Here's how the part is built. I have some questions about the finished solid (model axes, mm). Face numbers are marked on the shaded views. A direction names the side the tool comes from. Coordinates: 2 decimals unless noted, no trailing zeros. Write each loop counter-clockwise with the first axis right and the second up, starting at its lowest first coordinate (ties: lowest second). Pieces come first, ordered by that corner, then holes.
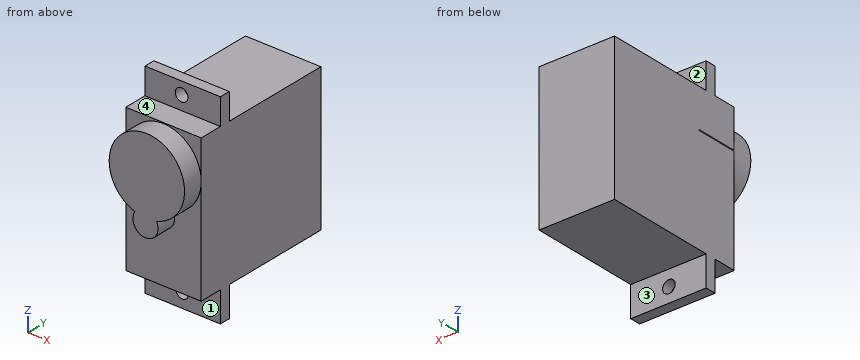
```python
from build123d import *

# Parameters (mm, degrees)
CYLINDER036_R             = 6
CYLINDER036_DEPTH         = 10
CYLINDER032_R             = 1
CYLINDER032_DEPTH         = 10
CYLINDER034_R             = 1
CYLINDER034_DEPTH         = 10
BOX003_W                  = 23
BOX003_H                  = 12
BOX003_DEPTH              = 23
BOX004_W                  = 32
BOX004_H                  = 12
BOX004_DEPTH              = 1.7
CYLINDER035_R             = 2
CYLINDER035_DEPTH         = 10
FUSION005_PITCH_ANGLE     = 90
FUSION005_PLACEMENT_ANGLE = -90


with BuildPart() as cylinder036:
    # Cylinder036 → Cylinder036 (new body)
    with BuildSketch(Plane(origin=(34.4857, 34.67, 6.56), x_dir=(1, 0, 0), z_dir=(0, 0, 1))):
        Circle(CYLINDER036_R)
    extrude(amount=CYLINDER036_DEPTH)


with BuildPart() as cylinder032:
    # Cylinder032 → Cylinder032 (new body)
    with BuildSketch(Plane(origin=(53.8219, 34.6, 2.58368), x_dir=(1, 0, 0), z_dir=(0, 0, 1))):
        Circle(CYLINDER032_R)
    extrude(amount=CYLINDER032_DEPTH)


with BuildPart() as cylinder034:
    # Cylinder034 → Cylinder034 (new body)
    with BuildSketch(Plane(origin=(26.1112, 34.5, 1.79316), x_dir=(1, 0, 0), z_dir=(0, 0, 1))):
        Circle(CYLINDER034_R)
    extrude(amount=CYLINDER034_DEPTH)


with BuildPart() as box003:
    # Box003 → Box003 (new body)
    with BuildSketch(Plane(origin=(28.340083, 28.670488, -9.643048), x_dir=(1, 0, 0), z_dir=(0, 0, 1))):
        with Locations((11.5, 6)):
            Rectangle(BOX003_W, BOX003_H)
    extrude(amount=BOX003_DEPTH)


with BuildPart() as cut039:
    # Box004 → Box004 (new body)
    with BuildSketch(Plane(origin=(24.149959, 28.670488, 7.966797), x_dir=(1, 0, 0), z_dir=(0, 0, 1))):
        with Locations((16, 6)):
            Rectangle(BOX004_W, BOX004_H)
    extrude(amount=BOX004_DEPTH)

    # Fusion003: union Box003
    add(box003.part)

    # Cut038: cut Cylinder034
    add(cylinder034.part, mode=Mode.SUBTRACT)

    # Cut039: cut Cylinder032
    add(cylinder032.part, mode=Mode.SUBTRACT)


with BuildPart() as fusion005:
    # Cylinder035 → Cylinder035 (new body)
    with BuildSketch(Plane(origin=(41.2515, 34.4472, 6.56), x_dir=(1, 0, 0), z_dir=(0, 0, 1))):
        Circle(CYLINDER035_R)
    extrude(amount=CYLINDER035_DEPTH)

    # Fusion005: union Cylinder036, Cut039
    add(cylinder036.part)
    add(cut039.part)


with BuildPart() as fusion005_1:
    # Fusion005 pitch: moved
    add(fusion005.part.rotate(Axis((0, 0, 0), (0, 1, 0)), FUSION005_PITCH_ANGLE))


with BuildPart() as fusion005_2:
    # Fusion005 placement: moved
    add(fusion005_1.part.moved(Location((-49, 17.44, 105.53))).rotate(Axis((-49, 17.44, 105.53), (0, 0, 1)), FUSION005_PLACEMENT_ANGLE))


solid = fusion005_2.part
```
1) I need wall thicknesses on probe 1 along Z at (x, y) = (-14.5, 8.6); probe 2 along Y at (x, z) = (-10.25, 61); probe 3 along Z at (x, y) = (-10.25, 13). Which ranges of each line are inside material? Lowest first, please.
Values follow:
probe 1: z = 49.38 to 50.71, 52.7 to 78.42, 80.42 to 81.38
probe 2: y = 4.08 to 27.08
probe 3: z = 54.19 to 77.19
2) Imagine slicing it at B-B on z = 63.5. Please give me the cut outline in (x, y).
Values follow:
outline: (-20.33, 4.08) - (-16.4, 4.08) - (-16.4, 0.88) - (-12.71, 0.88) - (-12.71, 4.08) - (-8.33, 4.08) - (-8.33, 27.08) - (-20.33, 27.08) - close
3) Imagine slicing it at A-A on x = -15. Please give me the cut outline in (y, z), then the cut area to 3 significant figures.
Values follow:
outline: (0.88, 62.33) - (4.08, 62.33) - (4.08, 54.19) - (7.77, 54.19) - (7.77, 52.51) - (9.47, 52.51) - (9.47, 54.19) - (27.08, 54.19) - (27.08, 77.19) - (9.47, 77.19) - (9.47, 78.55) - (7.77, 78.55) - (7.77, 77.19) - (4.08, 77.19) - (4.08, 77.01) - (0.88, 77.01) - close; (7.77, 49.38) - (9.47, 49.38) - (9.47, 50.91) - (7.77, 50.91) - close; (7.77, 80.28) - (9.47, 80.28) - (9.47, 81.38) - (7.77, 81.38) - close
area: 586 mm2
4) Imagine slicing it at C-C on y = 12. Please give me the cut outline in (x, z).
Values follow:
outline: (-20.33, 54.19) - (-8.33, 54.19) - (-8.33, 77.19) - (-20.33, 77.19) - close
5) Will these pins go through, and if not, where does the flat tip stop? pin 1 (3 mm diameter, centred on x = -14.5, y = 22, fed in from -Z); pin 2 (1.8 mm diameter, centred on x = -14.4, z = 51.71, fed in from +Y); pin 3 (1 mm diameter, centred on x = -13, y = 22, fed in from +Z); pin 4 (2.5 mm diameter, centred on x = -16, z = 51, fed in from -Y).
Values follow:
pin 1: stops at z = 54.19
pin 2: passes through
pin 3: stops at z = 77.19
pin 4: stops at y = 7.77
6) On a 3-axis mill with a long thin cutter (end or side, diameter ignored), from which of +Z, -Z, +X, -X, +Y, -Y can I reach the whole of each face in a straight line? I mean the marked faces 1, 2, 3 and 4. Say none if no direction works.
Values follow:
face 1: -Z, +X, -X, -Y
face 2: +Z, +X, -X, +Y
face 3: -Z, +X, -X, +Y
face 4: +Z, +X, -X, -Y
7) Imagine slicing it at D-D on x = -11. Please give me the cut outline in (y, z).
Values follow:
outline: (0.88, 66.05) - (4.08, 66.05) - (4.08, 54.19) - (7.77, 54.19) - (7.77, 49.38) - (9.47, 49.38) - (9.47, 54.19) - (27.08, 54.19) - (27.08, 77.19) - (9.47, 77.19) - (9.47, 81.38) - (7.77, 81.38) - (7.77, 77.19) - (4.08, 77.19) - (4.08, 76.04) - (0.88, 76.04) - close
